from build123d import *

# Parameters (mm, degrees)
CROQUIS1_W              = 49
CROQUIS1_H              = 73
CROQUIS1_R              = 8
CROQUIS1_R_2            = 2.5
CROQUIS1_W_2            = 12.5
CROQUIS1_H_2            = 22.9
SALIENTE_EXTRUIR4_DEPTH = 4
CROQUIS5_R              = 0.75
CORTAR_EXTRUIR1_DEPTH   = 4
CROQUIS7_W              = 49
CROQUIS7_H              = 5
SALIENTE_EXTRUIR5_DEPTH = 4
CROQUIS8_R              = 2.5
CORTAR_EXTRUIR2_DEPTH   = 10


with BuildPart() as part:
    # Croquis1 → Saliente-Extruir4 (new body)
    with BuildSketch(Plane(origin=(0, 0, 0), x_dir=(1, 0, 0), z_dir=(0, 1, 0))):
        with Locations((0, 0.5)):
            Rectangle(CROQUIS1_W, CROQUIS1_H)
        with Locations((14.5, -21.1)):
            Circle(CROQUIS1_R, mode=Mode.SUBTRACT)
        with Locations((-14.5, -21.1)):
            Circle(CROQUIS1_R, mode=Mode.SUBTRACT)
        with Locations((-14.5, 17)):
            Circle(CROQUIS1_R, mode=Mode.SUBTRACT)
        with Locations((14.5, 17)):
            Circle(CROQUIS1_R, mode=Mode.SUBTRACT)
        with Locations((-19.5, 32)):
            Circle(CROQUIS1_R_2, mode=Mode.SUBTRACT)
        with Locations((19.5, 32)):
            Circle(CROQUIS1_R_2, mode=Mode.SUBTRACT)
        with Locations((0, -17.55)):
            Rectangle(CROQUIS1_W_2, CROQUIS1_H_2, mode=Mode.SUBTRACT)
        with Locations((0, 20.55)):
            Rectangle(CROQUIS1_W_2, CROQUIS1_H_2, mode=Mode.SUBTRACT)
    extrude(amount=SALIENTE_EXTRUIR4_DEPTH)

    # Croquis5 → Cortar-Extruir1 (cut)
    with BuildSketch(Plane(origin=(0, 4, 0), x_dir=(1, 0, 0), z_dir=(0, 1, 0))):
        with Locations((0, 35)):
            Circle(CROQUIS5_R)
        with Locations((0, 6.1)):
            Circle(CROQUIS5_R)
        with Locations((0, -3.1)):
            Circle(CROQUIS5_R)
        with Locations((0, -32)):
            Circle(CROQUIS5_R)
    extrude(amount=-CORTAR_EXTRUIR1_DEPTH, mode=Mode.SUBTRACT)

    # Croquis7 → Saliente-Extruir5 (add)
    with BuildSketch(Plane(origin=(0, 4, 0), x_dir=(1, 0, 0), z_dir=(0, 1, 0))):
        with Locations((0, -38.5)):
            Rectangle(CROQUIS7_W, CROQUIS7_H)
    extrude(amount=-SALIENTE_EXTRUIR5_DEPTH)

    # Croquis8 → Cortar-Extruir2 (cut)
    with BuildSketch(Plane(origin=(0, 4, 0), x_dir=(1, 0, 0), z_dir=(0, 1, 0))):
        with Locations((-19.5, -36)):
            Circle(CROQUIS8_R)
        with Locations((19.5, -36)):
            Circle(CROQUIS8_R)
    extrude(amount=-CORTAR_EXTRUIR2_DEPTH, mode=Mode.SUBTRACT)


solid = part.part
Read the model definition and answer for the solid it produces. Units are mm, in the model's axes. A direction names the side the tool comes from. Round coordinates to 2 decimals unless told otherwise and drop trailing zeros. Write each loop counter-clockwise with the first axis right and the second up, starting at its lowest first coordinate (ties: lowest second). Pieces come first, ordered by that corner, then holes. Notation, with made-up numbers: M -20,-35 L 17,-35 A22 ccw 17,-4 Z; hole C 85.25,49 d2. An arc over 180 degrees is marked long. Use a Markdown table: item, result.
1) The part is cut by section C-C (z = 3.1). Write down the section's boundary in (x, y).
Answers follow:
| item | result |
|---|---|
| outline | M -24.5,0 L -0.75,0 L -0.75,4 L -24.5,4 Z; M 0.75,0 L 24.5,0 L 24.5,4 L 0.75,4 Z |
2) A flat-ended cylindrical pin translates along its axis: pin 1 (1.2 mm diameter, centred on x = 0, z = -6.1, fed in from +Y). Find the tip coordinate at first contact, or state that the pin passes through.
Answers follow:
| item | result |
|---|---|
| pin 1 | passes through |
3) The part is cut by section D-D (x = 0). Write down the section's boundary in (y, z), plus the area to 3 significant figures.
Answers follow:
| item | result |
|---|---|
| outline | M 0,-37 L 4,-37 L 4,-35.75 L 0,-35.75 Z; M 0,-34.25 L 4,-34.25 L 4,-32 L 0,-32 Z; M 0,-9.1 L 4,-9.1 L 4,-6.85 L 0,-6.85 Z; M 0,-5.35 L 4,-5.35 L 4,2.35 L 0,2.35 Z; M 0,3.85 L 4,3.85 L 4,6.1 L 0,6.1 Z; M 0,29 L 4,29 L 4,31.25 L 0,31.25 Z; M 0,32.75 L 4,32.75 L 4,41 L 0,41 Z |
| area | 105 mm2 |
4) A tool of negligible diameter and unlimited length cuts with its end or side. For faces 5 (the flat face through (0, 2, 41)), 6 (the flat face through (-6.25, 2, 18)), from which of +Z, -Z, +X, -X, +Y, -Y can it reach the whole face along a straight path? Write none if from no direction.
Answers follow:
| item | result |
|---|---|
| face 5 | +Z, +X, -X, +Y, -Y |
| face 6 | +Y, -Y |
5) For a pull along X with two mould halves and no side action, classify faces 1 (the flat face through (-24.5, 2, 3)), 2 (the flat face through (24.5, 2, 3)), 3 (the flat face through (0, 2, -9.1)), 4 (the flat face through (0, 4, 1)) as pulls with the +X half, pulls with the -X half, needs draft (parallel to the pull), parting line crosses it, or undercut.
Answers follow:
| item | result |
|---|---|
| face 1 | pulls with the -X half |
| face 2 | pulls with the +X half |
| face 3 | undercut |
| face 4 | needs draft |
6) The part is cut by section B-B (z = 36). Write down the section's boundary in (x, y), plus the area to 3 significant figures.
Answers follow:
| item | result |
|---|---|
| outline | M -24.5,0 L -22,0 L -22,4 L -24.5,4 Z; M -17,0 L 17,0 L 17,4 L -17,4 Z; M 22,0 L 24.5,0 L 24.5,4 L 22,4 Z |
| area | 156 mm2 |
7) Straight lines are drawn through the part: line 1 along Z through (x, y) = (14.5, 0.55); line 2 along Z through (x, y) = (-4, 3.15); line 3 along X through (y, z) = (2.6, -23). For each, find the intervals that lie inside material, in ascending order. Write a range as [from, to].
Answers follow:
| item | result |
|---|---|
| line 1 | z = [-37, -25], [-9, 13.1], [29.1, 41] |
| line 2 | z = [-37, -32], [-9.1, 6.1], [29, 41] |
| line 3 | x = [-24.5, -19.79], [-9.21, -6.25], [6.25, 9.21], [19.79, 24.5] |
8) The part is cut by section A-A (x = 14.5). Write down the section's boundary in (y, z), plus the area to 3 significant figures.
Answers follow:
| item | result |
|---|---|
| outline | M 0,-37 L 4,-37 L 4,-25 L 0,-25 Z; M 0,-9 L 4,-9 L 4,13.1 L 0,13.1 Z; M 0,29.1 L 4,29.1 L 4,41 L 0,41 Z |
| area | 184 mm2 |
